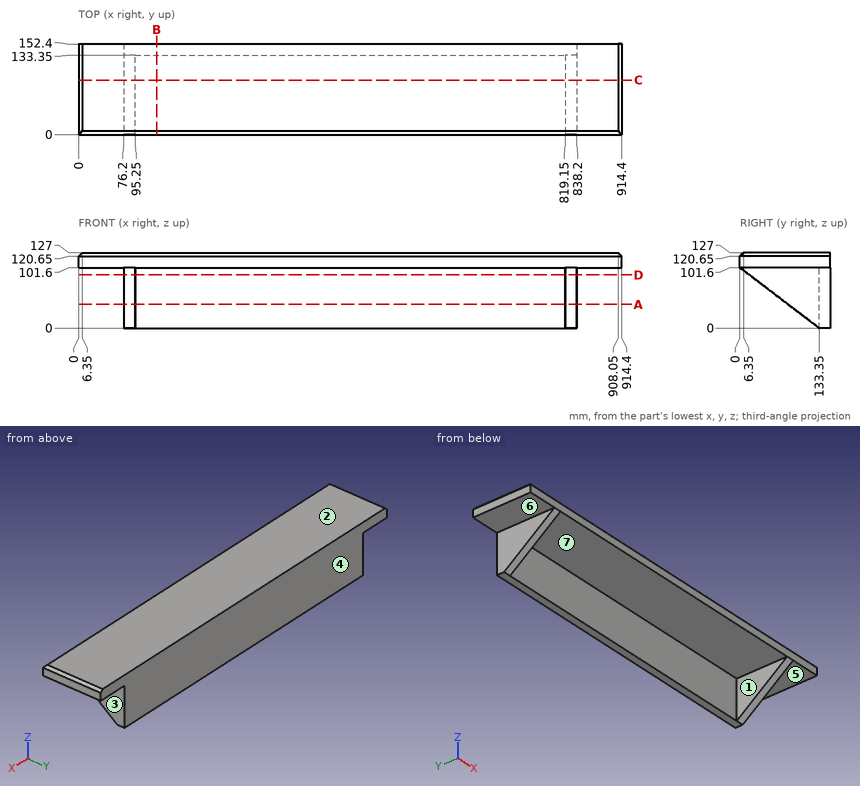
For this review, use the dimensioned drawing (mm, ordinates from the lowest corner) and the shaded views. A direction names the side the tool comes from. Give positions to 0.01 mm unless a question says otherwise; leave off trailing zeros. Order: outer loops, then holes, each group sorted by start corner. A loop starts at its lowest first (then second) coordinate and runs counter-clockwise, first axis right, second up.
1. To check wall thickness, follow L1, parallel to X at y = 68.5, z = 87; L2, parallel to Z at x = 252.5, y = 77. State the ranges of each line that lie inside material, in increasing order.
Solution:
L1: x = 76.2 to 95.25, 819.15 to 838.2
L2: z = 101.6 to 127
2. Add section A-A, the plane z = 40. State the section outline as (x, y) points.
Solution:
outline: (76.2, 80.85) - (95.25, 80.85) - (95.25, 133.35) - (819.15, 133.35) - (819.15, 80.85) - (838.2, 80.85) - (838.2, 152.4) - (76.2, 152.4) - close
3. For pin 1 Ø23 at (x, y) = (20, 51.5) entering from -Z; pin 2 Ø5 at (x, z) = (663.5, 29.5) entering from -Y, all flat-tipped, find the tip position at first contact; note any pin that passes through.
Solution:
pin 1: stops at z = 101.6
pin 2: stops at y = 133.35
4. Add section D-D, the plane z = 89.5. State the section outline as (x, y) points.
Solution:
outline: (76.2, 15.88) - (95.25, 15.88) - (95.25, 133.35) - (819.15, 133.35) - (819.15, 15.88) - (838.2, 15.88) - (838.2, 152.4) - (76.2, 152.4) - close
5. Add section B-B, the plane x = 131.5. State the section outline as (y, z) points.
Solution:
outline: (0, 101.6) - (133.35, 101.6) - (133.35, 0) - (152.4, 0) - (152.4, 127) - (6.35, 127) - (0, 120.65) - close
6. Tool access review of the marked faces 4, 5, 6 and 7: name each direction out of +Z, -Z, +X, -X, +Y, -Y from which nothing blocks a thin tool from reaching the whole face with its end or side.
Solution:
face 4: +Z, -Z, +X, -X, +Y
face 5: -Z, +X, +Y, -Y
face 6: -Z, -X, +Y, -Y
face 7: -Z, -Y
7. Add section C-C, the plane y = 91.5. State the section outline as (x, z) points.
Solution:
outline: (0, 101.6) - (76.2, 101.6) - (76.2, 31.89) - (95.25, 31.89) - (95.25, 101.6) - (819.15, 101.6) - (819.15, 31.89) - (838.2, 31.89) - (838.2, 101.6) - (914.4, 101.6) - (914.4, 120.65) - (908.05, 127) - (6.35, 127) - (0, 120.65) - close
8. Mouldability with a two-part tool opening along X and no side actions: class the marked faces 1, 2 and 3 as +X half, -X half, draft (parallel to the pull), parting line (faces both ways), or undercut.
Solution:
face 1: undercut
face 2: draft
face 3: +X half
